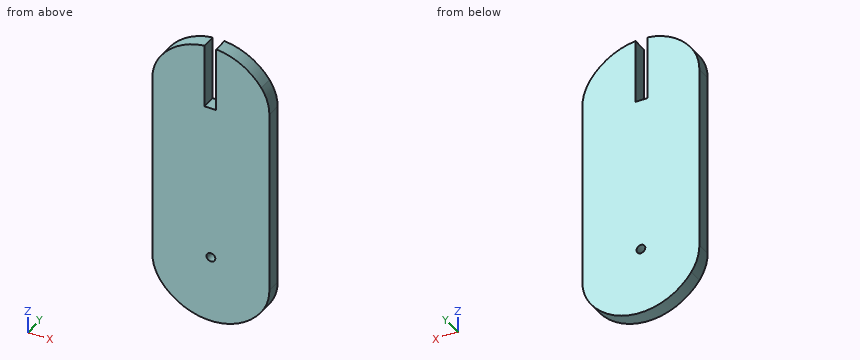
from build123d import *

# Parameters (mm, degrees)
SKETCH2_W           = 40
SKETCH2_H           = 70
BOSS_EXTRUDE1_DEPTH = 5
FILLET1_R           = 15
CUT_EXTRUDE1_DEPTH  = 6
SKETCH4_R           = 1.5
CUT_EXTRUDE2_DEPTH  = 6


with BuildPart() as part:
    # Sketch2 → Boss-Extrude1 (new body)
    with BuildSketch(Plane(origin=(0, 0, 0), x_dir=(1, 0, 0), z_dir=(0, 1, 0))):
        with BuildLine():
            Line((-20, -35), (20, -35))
            ThreePointArc((20, -35), (0, -49.312603136), (-20, -35))
        make_face()
        Rectangle(SKETCH2_W, SKETCH2_H)
        with BuildLine():
            ThreePointArc((-20, 35), (0, 49.305454963), (20, 35))
            Line((20, 35), (-20, 35))
        make_face()
    extrude(amount=BOSS_EXTRUDE1_DEPTH)

    # Fillet1
    fillet1_edges = [part.edges().sort_by_distance(p)[0] for p in [
        (-20, 2.5, 35),
        (-20, 2.5, -35),
        (20, 2.5, -35),
        (20, 2.5, 35),
    ]]
    fillet(fillet1_edges, radius=FILLET1_R)

    # Sketch3 → Cut-Extrude1 (cut, through all)
    with BuildSketch(Plane.XZ):
        Polygon((0, 49.312603136), (1.823748233, 49.312603136), (1.823748233, 27.312603136), (-2.176251767, 27.312603136), (-2.176251767, 49.312603136), align=None)
    extrude(amount=-CUT_EXTRUDE1_DEPTH, mode=Mode.SUBTRACT)

    # Sketch4 → Cut-Extrude2 (cut, through all)
    with BuildSketch(Plane.XZ):
        with Locations((0, -26.387396864)):
            Circle(SKETCH4_R)
    extrude(amount=-CUT_EXTRUDE2_DEPTH, mode=Mode.SUBTRACT)


solid = part.part
Verification items for the finished model (mm, model axes). Coordinates: 2 decimals unless noted, no trailing zeros. Loops run counter-clockwise (first coordinate to the right, second up) from the corner with the lowest first, then second, coordinate; pieces in that order, holes last. Notation, with made-up numbers: (3.5, 82) -> (12.5, 82) arc R11 ccw to (12.5, 86) -> close; hole circle Ø3 at (63, -18). An arc over 180 degrees is marked (long way). Write each question's results on one line, items separated by ' | '.
Item 1: Section check B-B, the plane x = 0. Enter the section's corners in (y, z), plus the area to 3 significant figures.
Found:
outline: (0, -49.31) -> (5, -49.31) -> (5, -27.89) -> (0, -27.89) -> close; (0, -24.89) -> (5, -24.89) -> (5, 27.31) -> (0, 27.31) -> close | area: 368 mm2
Item 2: Material ranges on L1, parallel to X at y = 1.1, z = 29.5; L2, parallel to X at y = 2.85, z = 45; L3, parallel to Z at x = -5, y = 4.6, recorded low to high.
Found:
L1: x = -20 to -2.18, 1.82 to 20 | L2: x = -12.79 to -2.18, 1.82 to 12.79 | L3: z = -48.71 to 48.71
Item 3: Section check C-C, the plane y = 3.4. Enter the section's corners in (x, z).
Found:
outline: (-20, -31.72) arc R15 ccw to (-17.23, -40.41) arc R21.13 ccw to (17.23, -40.41) arc R15 ccw to (20, -31.72) -> (20, 31.73) arc R15 ccw to (17.23, 40.41) arc R21.13 ccw to (1.82, 49.23) -> (1.82, 27.31) -> (-2.18, 27.31) -> (-2.18, 49.2) arc R21.13 ccw to (-17.23, 40.41) arc R15 ccw to (-20, 31.73) -> close; hole circle Ø3 at (0, -26.39)
Item 4: Section check D-D, the plane x = -16. Enter the section's corners in (y, z), plus the area to 3 significant figures.
Found:
outline: (0, -41.98) -> (5, -41.98) -> (5, 41.98) -> (0, 41.98) -> close | area: 420 mm2
Item 5: Section check A-A, the plane z = 30. Enter the section's corners in (x, y).
Found:
outline: (-20, 0) -> (-2.18, 0) -> (-2.18, 5) -> (-20, 5) -> close; (1.82, 0) -> (20, 0) -> (20, 5) -> (1.82, 5) -> close
Item 6: Gauge pin test, flat ends, axial feed: pin 1 (1.2 mm diameter, centred on x = 1, y = 3.5, fed in from +Z); pin 2 (3 mm diameter, centred on x = 12.5, y = 2.5, fed in from -Z). Record the tip position at first contact, or that the pin passes through.
Found:
pin 1: stops at z = 27.31 | pin 2: stops at z = -46.22
